from build123d import *

# Parameters (mm, degrees)
PAD001_DEPTH       = 6
POLARPATTERN_COUNT = 6


with BuildPart() as part:
    # Sketch (on XZ_Plane of Origin) → Revolution (revolve)
    with BuildSketch(Plane.XZ):
        with BuildLine():
            Line((0, 32), (0, 21))
            ThreePointArc((0, 21), (-12.020815, 16.020815), (-17, 4))
            Line((-17, 0), (-17, 4))
            Line((-20, 0), (-17, 0))
            Line((-20, 4), (-20, 0))
            ThreePointArc((-12, 20), (-17.888544, 12.944272), (-20, 4))
            Line((-12, 20), (-12, 32))
            Line((-12, 32), (0, 32))
        make_face()
    revolve(axis=Axis((0, 0, 0), (0, 0, 1)))

    # Sketch001 (on Face2 of Revolution) → Pad001 (new body)
    with BuildSketch(Plane.XY.offset(32)):
        with BuildLine():
            ThreePointArc((0, 13.5), (2.90558, 13.757845), (5.72035, 14.523321))
            ThreePointArc((9.71739, 12.215628), (8.260413, 14.307455), (5.72035, 14.523321))
            ThreePointArc((9.71739, 12.215628), (10.461853, 9.395229), (11.691343, 6.75))
            Line((0, 0), (11.691343, 6.75))
            Line((0, 13.5), (0, 0))
        make_face()
    pad001 = extrude(amount=PAD001_DEPTH)

    # PolarPattern: Pad001 ×6 about axis
    polarpattern_axis = Axis((0, 0, 32), (0, 0, 1))
    for i in range(1, POLARPATTERN_COUNT):
        add(pad001.rotate(polarpattern_axis, i * 360 / POLARPATTERN_COUNT))


solid = part.part
Read the model definition and answer for the solid it produces. Units are mm, in the model's axes. A direction names the side the tool comes from. Coordinates: 2 decimals unless noted, no trailing zeros. Loops run counter-clockwise (first coordinate to the right, second up) from the corner with the lowest first, then second, coordinate; pieces in that order, holes last. Notation, with made-up numbers: (59, 57.5) -> (102, 57.5) arc R15 cw to (102, 64.5) -> close; hole circle Ø7 at (14, -27). An arc over 180 degrees is marked (long way). Answer in a Markdown table with one row per item.
Item 1: Each of these flat-tipped pins is pushed along its axis until it touches: P1, Ø10, axis at y = 0, z = 29.5, coming from the +X side; P2, Ø2, axis at x = 0, y = -3, coming from the -Z side; P3, Ø6, axis at y = -7, z = 22.5, coming from the -X side. Where does it stop, or does it pass through?
Returned:
| item | result |
|---|---|
| P1 | stops at x = 16.52 |
| P2 | stops at z = 20.52 |
| P3 | stops at x = -11.31 |
Item 2: Straight lines are drawn through the part: line 1 along X through (y, z) = (0, 2.6); line 2 along X through (y, z) = (0, 31.5). For each, find the intervals that lie inside material, in ascending order. Write a range as [from, to].
Returned:
| item | result |
|---|---|
| line 1 | x = [-20, -17], [17, 20] |
| line 2 | x = [-12, 12] |
Item 3: For a pull along Z with two mould halves and no side action, classify faces 1 (the flat face through (9, 15, 0)), 2 (the cylindrical face through (4.336, 19.524, 1.972)), 3 (the cylindrical face through (11.99, -0.53, 26.08)) as released by +Z, released by -Z, zero draft, split by the parting line, or undercut.
Returned:
| item | result |
|---|---|
| face 1 | released by -Z |
| face 2 | zero draft |
| face 3 | undercut |
Item 4: A cutting plane is placed at A-A on z = 27. Determine the outline of the cut face in (x, y), plus the area to 3 significant figures.
Returned:
| item | result |
|---|---|
| outline | circle Ø24 at (0, 0) |
| area | 452 mm^2 |
Item 5: For faces 4 (the cylindrical face through (16.52, -0.04, 34.96)), 5 (the cylindrical face through (-9.139, -14.334, 2.028)), 6 (the cylindrical face through (8.228, -14.326, 34.958)), 7 (the cylindrical face through (-16.52, 0.04, 34.96)), determine the directions among +Z, -Z, +X, -X, +Y, -Y from which every point of the face is accessible in a straight line to the end or side of a thin tool.
Returned:
| item | result |
|---|---|
| face 4 | +Z, +X |
| face 5 | -Z |
| face 6 | +Z, -Y |
| face 7 | +Z, -X |
